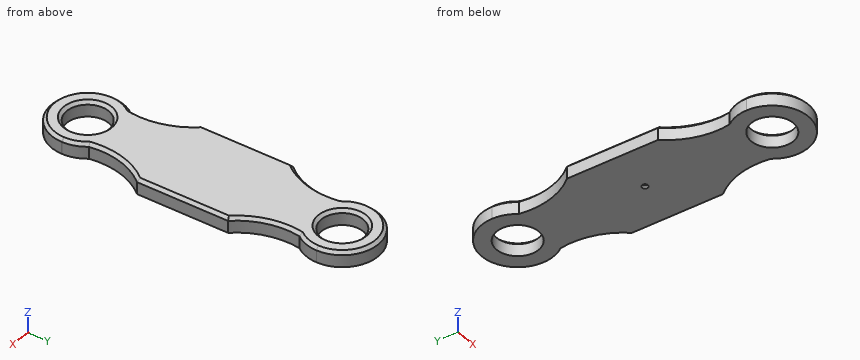
from build123d import *

# Parameters (mm, degrees)
F0_W        = 19.05
F0_H        = 19.05
F0_R        = 0.635
F0_R_2      = 4.445
F1_DEPTH    = 3.175
F2_C1_SIZE  = 0.635
F2_C2_SIZE  = 0.635
F2_C3_SIZE  = 0.635
F2_C4_SIZE  = 0.635
F2_C5_SIZE  = 0.635
F2_C6_SIZE  = 0.635
F2_C7_SIZE  = 0.635
F2_C8_SIZE  = 0.635
F2_C9_SIZE  = 0.6349
F2_C10_SIZE = 0.6349
F3_DEPTH    = 0.635


# Not quite as in the source:
# - a fillet or chamfer is up to 0.001 mm smaller than in the source, because OpenCascade refuses the exact size


with BuildPart() as f1:
    # F0 (on Top) → F1 (new body)
    with BuildSketch(Plane.XY):
        Rectangle(F0_W, F0_H)
        Circle(F0_R, mode=Mode.SUBTRACT)
        with BuildLine():
            Line((9.525, -9.525), (-9.525, -9.525))
            ThreePointArc((-9.525, -9.525), (-6.3836187271, -15.3786997104), (-6.0310725347, -22.012687032))
            ThreePointArc((-6.0310725347, -22.012687032), (0.0350329382, -19.0500805324), (6.0736411029, -22.0683390224))
            ThreePointArc((6.0736411029, -22.0683390224), (6.3936440411, -15.409890989), (9.525, -9.525))
        make_face()
        with BuildLine():
            ThreePointArc((6.0736411029, -22.0683390224), (0.0350329382, -19.0500805324), (-6.0310725347, -22.012687032))
            ThreePointArc((-6.0310725347, -22.012687032), (-6.6363180101, -24.4058987838), (-7.62, -26.67))
            ThreePointArc((-7.62, -26.67), (0, -34.29), (7.62, -26.67))
            ThreePointArc((7.62, -26.67), (7.619882327, -26.6276523681), (7.6195293118, -26.5853060441))
            ThreePointArc((7.6195293118, -26.5853060441), (6.6686101992, -24.3877327559), (6.0736411029, -22.0683390224))
        make_face()
        with Locations((0, -26.67)):
            Circle(F0_R_2, mode=Mode.SUBTRACT)
        with BuildLine():
            ThreePointArc((-7.62, -26.67), (-6.6363180101, -24.4058987838), (-6.0310725347, -22.012687032))
            ThreePointArc((-6.0310725347, -22.012687032), (-7.2118365454, -24.2095501137), (-7.62, -26.67))
        make_face()
        with BuildLine():
            ThreePointArc((7.6195293118, -26.5853060441), (7.2094713239, -24.202628275), (6.0736411029, -22.0683390224))
            ThreePointArc((6.0736411029, -22.0683390224), (6.6686101992, -24.3877327559), (7.6195293118, -26.5853060441))
        make_face()
        with BuildLine():
            ThreePointArc((-6.0736411029, 22.0683390224), (-6.3936440411, 15.409890989), (-9.525, 9.525))
            Line((-9.525, 9.525), (9.525, 9.525))
            ThreePointArc((9.525, 9.525), (6.3836187271, 15.3786997104), (6.0310725347, 22.012687032))
            ThreePointArc((6.0310725347, 22.012687032), (-0.0350329382, 19.0500805324), (-6.0736411029, 22.0683390224))
        make_face()
        with BuildLine():
            ThreePointArc((-7.6195293118, 26.5853060441), (-6.6686101992, 24.3877327559), (-6.0736411029, 22.0683390224))
            ThreePointArc((-6.0736411029, 22.0683390224), (-0.0350329382, 19.0500805324), (6.0310725347, 22.012687032))
            ThreePointArc((6.0310725347, 22.012687032), (6.6363180101, 24.4058987838), (7.62, 26.67))
            ThreePointArc((7.62, 26.67), (-0.0423476319, 34.289882327), (-7.6195293118, 26.5853060441))
        make_face()
        with Locations((0, 26.67)):
            Circle(F0_R_2, mode=Mode.SUBTRACT)
        with BuildLine():
            ThreePointArc((-7.6195293118, 26.5853060441), (-7.2094713239, 24.202628275), (-6.0736411029, 22.0683390224))
            ThreePointArc((-6.0736411029, 22.0683390224), (-6.6686101992, 24.3877327559), (-7.6195293118, 26.5853060441))
        make_face()
        with BuildLine():
            ThreePointArc((7.62, 26.67), (6.6363180101, 24.4058987838), (6.0310725347, 22.012687032))
            ThreePointArc((6.0310725347, 22.012687032), (7.2118365454, 24.2095501137), (7.62, 26.67))
        make_face()
        Circle(F0_R)
    extrude(amount=F1_DEPTH)

    # F2: chamfer of 0.635 on 10 edges, made by hand

    # F2_c1
    f2_c1_edges = [f1.edges().sort_by_distance(p)[0] for p in [
        (-9.525, 0, 3.175),
    ]]
    chamfer(f2_c1_edges, length=F2_C1_SIZE)

    # F2_c2
    f2_c2_edges = [f1.edges().sort_by_distance(p)[0] for p in [
        (-6.2554888364, -15.867774564, 3.175),
    ]]
    chamfer(f2_c2_edges, length=F2_C2_SIZE)

    # F2_c3
    f2_c3_edges = [f1.edges().sort_by_distance(p)[0] for p in [
        (6.3936440411, -15.409890989, 3.175),
    ]]
    chamfer(f2_c3_edges, length=F2_C3_SIZE)

    # F2_c4
    f2_c4_edges = [f1.edges().sort_by_distance(p)[0] for p in [
        (9.525, 0.4748240758, 3.175),
    ]]
    chamfer(f2_c4_edges, length=F2_C4_SIZE)

    # F2_c5
    f2_c5_edges = [f1.edges().sort_by_distance(p)[0] for p in [
        (6.2554888364, 15.867774564, 3.175),
    ]]
    chamfer(f2_c5_edges, length=F2_C5_SIZE)

    # F2_c6
    f2_c6_edges = [f1.edges().sort_by_distance(p)[0] for p in [
        (-6.2671958343, 15.9012829536, 3.175),
    ]]
    chamfer(f2_c6_edges, length=F2_C6_SIZE)

    # F2_c7
    f2_c7_edges = [f1.edges().sort_by_distance(p)[0] for p in [
        (-4.445, -26.67, 3.175),
    ]]
    chamfer(f2_c7_edges, length=F2_C7_SIZE)

    # F2_c8
    f2_c8_edges = [f1.edges().sort_by_distance(p)[0] for p in [
        (-4.445, 26.67, 3.175),
    ]]
    chamfer(f2_c8_edges, length=F2_C8_SIZE)

    # F2_c9 (size 0.635 in the source; OpenCascade refuses exactly that, so slightly less here)
    f2_c9_edges = [f1.edges().sort_by_distance(p)[0] for p in [
        (-0.0350329382, -34.2899194676, 3.175),
    ]]
    chamfer(f2_c9_edges, length=F2_C9_SIZE)

    # F2_c10 (size 0.635 in the source; OpenCascade refuses exactly that, so slightly less here)
    f2_c10_edges = [f1.edges().sort_by_distance(p)[0] for p in [
        (0.0350329382, 34.2899194676, 3.175),
    ]]
    chamfer(f2_c10_edges, length=F2_C10_SIZE)

    # F0 (on Top) → F3 (cut)
    with BuildSketch(Plane.XY):
        Circle(F0_R)
    extrude(amount=F3_DEPTH, mode=Mode.SUBTRACT)


solid = f1.part
Check sheet for the modelled part. Datum: model origin and axes. Units: mm. Give positions to 0.01 mm unless a question says otherwise; leave off trailing zeros. Order: outer loops, then holes, each group sorted by start corner. A loop starts at its lowest first (then second) coordinate and runs counter-clockwise, first axis right, second up. Notation, with made-up numbers: (23.5, -9) - (55.5, -9) arc R10 ccw to (55.5, -1) - close; hole circle Ø4 at (31.25, 23.5). An arc over 180 degrees is marked (long way). Answer as CSV lines item,"result".
1. Section check B-B (z = 1.3). Record the boundary of the cut face in (x, y) (3 decimals).
Result sheet:
outline,"(-9.525, -9.525) arc R15.24 cw to (-6.031, -22.013) arc R7.62 ccw (long way) to (7.62, -26.67) arc R7.62 ccw to (7.62, -26.585) arc R7.62 ccw to (6.074, -22.068) arc R15.24 cw to (9.525, -9.525) - (9.525, 9.525) arc R15.24 cw to (6.031, 22.013) arc R7.62 ccw (long way) to (-6.074, 22.068) arc R15.24 cw to (-9.525, 9.525) - close; hole circle Ø8.89 at (0, -26.67); hole circle Ø8.89 at (0, 26.67)"
2. Scan lines: probe 1 along Y at (x, z) = (0, 2) (3 decimals); probe 2 along Y at (x, z) = (0, 0.35) (3 decimals); probe 3 along Y at (x, z) = (1, 0.85). Record each from-to range of solid material in increasing order. Write a range as from..to.
Result sheet:
probe 1,"-34.29..-31.115, -22.225..22.225, 31.115..34.29"
probe 2,"-34.29..-31.115, -22.225..-0.635, 0.635..22.225, 31.115..34.29"
probe 3,"-34.22..-31, -22.34..22.34, 31..34.22"
3. Go/stop test with flat-tipped pins: P1, Ø7, axis at x = 0, y = 26.67, coming from the +Z side; P2, Ø1, axis at x = -5.5, z = 1, coming from the +Y side; P3, Ø1, axis at x = 2, z = 1.5, coming from the -Y side; P4, Ø1, axis at x = 0, y = 0, coming from the -Z side (3 decimals). Record where each tip stops, or that it passes through.
Result sheet:
P1,"through"
P2,"y = 32.42"
P3,"y = -34.14"
P4,"z = 0.635"
4. Section check A-A (x = 0). Record the boundary of the cut face in (y, z) (3 decimals).
Result sheet:
outline,"(-34.29, 0) - (-31.115, 0) - (-31.115, 2.54) - (-31.75, 3.175) - (-33.655, 3.175) - (-34.29, 2.54) - close; (-22.225, 0) - (-0.635, 0) - (-0.635, 0.635) - (0.635, 0.635) - (0.635, 0) - (22.225, 0) - (22.225, 2.54) - (21.59, 3.175) - (-21.59, 3.175) - (-22.225, 2.54) - close; (31.115, 0) - (34.29, 0) - (34.29, 2.54) - (33.655, 3.175) - (31.75, 3.175) - (31.115, 2.54) - close"
